```python
from build123d import *

# Parameters (mm, degrees)
SKETCH1_W                         = 25.4
SKETCH1_H                         = 12.7
EXTRUDE1_DEPTH                    = 22.86
F_1_4_CLEARANCE_HOLE1_D           = 6.7564
F_1_4_CLEARANCE_HOLE1_ON_FACE_2_D = 6.7564


with BuildPart() as part:
    # Sketch1 → Extrude1 (new body)
    with BuildSketch(Plane.XY):
        Rectangle(SKETCH1_W, SKETCH1_H)
    extrude(amount=EXTRUDE1_DEPTH)

    # 1/4 Clearance Hole1 (through all)
    with Locations(Plane(origin=(0, 0, 0), x_dir=(-1, 0, 0), z_dir=(0, 0, -1))):
        with Locations((0, 0)):
            Hole(F_1_4_CLEARANCE_HOLE1_D / 2)

    # 1/4 Clearance Hole1 on face 2 (through all)
    with Locations(Plane.XY.offset(22.86)):
        with Locations((0, 0)):
            Hole(F_1_4_CLEARANCE_HOLE1_ON_FACE_2_D / 2)


solid = part.part
```
Work out the finished part from the listing and answer in its coordinate system (mm). Coordinates: 2 decimals unless noted, no trailing zeros. Write each loop counter-clockwise with the first axis right and the second up, starting at its lowest first coordinate (ties: lowest second). Pieces come first, ordered by that corner, then holes.
Q1. A cutting plane is placed at A-A, the plane y = 0. Give the vertices of the cut face in (x, z), then the cut area to 3 significant figures.
Q2. A cutting plane is placed at B-B, the plane z = 5. Give the vertices of the cut face in (x, y).
Q3. Each of these flat-tipped pins is pushed along its axis until it touches: pin 1 Ø6 at (x, y) = (0, 0) entering from -Z; pin 2 Ø2 at (x, y) = (0.5, -2.5) entering from +Z. Where does it stop, or does it pass through?
Q4. A cutting plane is placed at C-C, the plane x = 0. Give the vertices of the cut face in (y, z), then the cut area to 3 significant figures.
Q5. Determine the mould class of faces 1 (the face through (12.7, 0, 11)), 2 (the face through (-2.681, -2.056, 11.59)), 3 (the face through (3, -3, 0)) for opening direction X: released by +X, released by -X, zero draft, split by the parting line, or undercut.
Q6. Find the intervals of material crossed by line 1 (Y direction, x = 0, z = 5.25); line 2 (X direction, y = 0, z = 9); line 3 (X direction, y = 0.5, z = 17.25), in increasing order.
Findings below:
1. outline: (-12.7, 0) - (-3.38, 0) - (-3.38, 22.86) - (-12.7, 22.86) - close; (3.38, 0) - (12.7, 0) - (12.7, 22.86) - (3.38, 22.86) - close
1. area: 426 mm2
2. outline: (-12.7, -6.35) - (12.7, -6.35) - (12.7, 6.35) - (-12.7, 6.35) - close; hole circle Ø6.76 at (0, 0)
3. pin 1: passes through
3. pin 2: stops at z = 22.86
4. outline: (-6.35, 0) - (-3.38, 0) - (-3.38, 22.86) - (-6.35, 22.86) - close; (3.38, 0) - (6.35, 0) - (6.35, 22.86) - (3.38, 22.86) - close
4. area: 136 mm2
5. face 1: released by +X
5. face 2: undercut
5. face 3: zero draft
6. line 1: y = -6.35 to -3.38, 3.38 to 6.35
6. line 2: x = -12.7 to -3.38, 3.38 to 12.7
6. line 3: x = -12.7 to -3.34, 3.34 to 12.7
